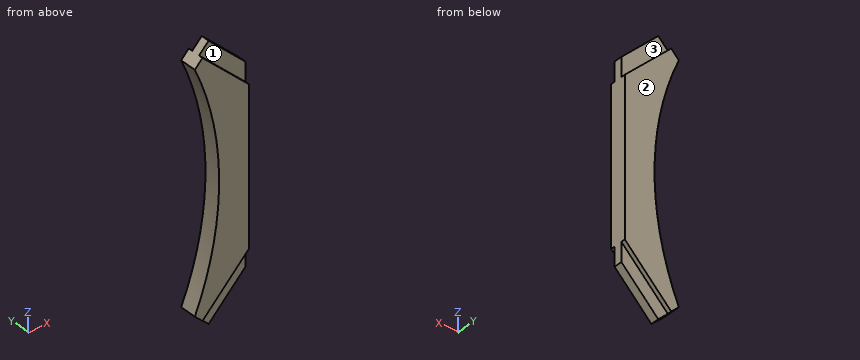
```python
from build123d import *

# Parameters (mm, degrees)
F1_DEPTH = 38.1
F2_DEPTH = 19.05


with BuildPart() as f1:
    # F0 (on Front) → F1 (new body, symmetric)
    with BuildSketch(Plane.XZ):
        with BuildLine():
            Line((127, 289.350816), (-127, 543.350816))
            ThreePointArc((-127, 543.350816), (-12.7, -4.446916), (-127, -552.244648))
            Line((-127, -552.244648), (127, -298.244648))
            Line((127, -298.244648), (127, 289.350816))
        make_face()
        Polygon((127, -298.244648), (-127, -552.244648), (-100.059232, -579.185416), (127, -352.126184), align=None)
        Polygon((-100.059232, 570.291584), (-127, 543.350816), (127, 289.350816), (127, 343.232352), align=None)
        Polygon((-91.078976, 579.27184), (-100.059232, 570.291584), (127, 343.232352), (127, 361.192865), align=None)
        Polygon((127, -352.126184), (-100.059232, -579.185416), (-91.078976, -588.165672), (127, -370.086696), align=None)
    extrude(amount=F1_DEPTH, both=True)

    # F0 (on Front) → F2 (join, symmetric)
    with BuildSketch(Plane.XZ):
        Polygon((127, 361.192865), (127, 450.995426), (-46.177695, 624.173121), (-91.078976, 579.27184), align=None)
        Polygon((127, -370.086696), (-91.078976, -588.165672), (-46.177695, -633.066953), (127, -459.889258), align=None)
    extrude(amount=F2_DEPTH, both=True)


solid = f1.part
```
Source: CAD feature listing. Evaluate the final solid. Frame: model axes, mm. Face numbers are marked on the shaded views. A direction names the side the tool comes from. Round coordinates to 2 decimals unless told otherwise and drop trailing zeros. Write each loop counter-clockwise with the first axis right and the second up, starting at its lowest first coordinate (ties: lowest second). Pieces come first, ordered by that corner, then holes. Notation, with made-up numbers: M 88.25,3 L 130.25,3 A23 cw 130.25,27 Z; hole C 53.5,24.5 d11. An arc over 180 degrees is marked long. Answer as a JSON object with one key per item and string values. Group by question number.
(1) Section query B-B on y = -8. Output: boundary loops of the cut face in (x, z).
(2) First-contact query: pin 1 (12 mm diameter, centred on y = 2.5, z = 291, fed in from -X); pin 2 (2 mm diameter, centred on x = 97.5, z = -449.5, fed in from +Y); pin 3 (3 mm diameter, centred on x = 87, y = -29.5, fed in from +Z). Flat tips, straight axial feed; report the tip coordinate or a pass-through.
(3) Section query D-D on x = 60. Output: boundary loops of the cut face in (y, z).
(4) Reachability of the marked faces 1, 2 and 3 from +Z, -Z, +X, -X, +Y, -Y: full face, straight path, thin tool, end or side. Return the list, or none.
(5) Section query A-A on x = -73.5. Output: boundary loops of the cut face in (y, z), then the cut area to 3 significant figures.
(6) Section query C-C on z = -532.5. Output: boundary loops of the cut face in (x, y).
(7) Ray query, line 1 (X direction, y = -17.5, z = -23); line 2 (Z direction, x = 34, y = -22); line 3 (X direction, y = -31, z = 145). Return the intervals inside material, ascending. Write a range as [from, to].
Computed values:
{
 "1": {"outline": "M -127,-552.24 L -46.18,-633.07 L 127,-459.89 L 127,451 L -46.18,624.17 L -127,543.35 A1369.85 cw Z"},
 "2": {"pin 1": "x = -46.28", "pin 2": "y = 19.05", "pin 3": "z = 402.69"},
 "3": {"outline": "M -38.1,-437.09 L -19.05,-437.09 L -19.05,-526.89 L 19.05,-526.89 L 19.05,-437.09 L 38.1,-437.09 L 38.1,428.19 L 19.05,428.19 L 19.05,518 L -19.05,518 L -19.05,428.19 L -38.1,428.19 Z"},
 "4": {"face 1": "+Z, +X, -Y", "face 2": "+Z, -Z, +X, -X, +Y", "face 3": "+Z, +X, +Y"},
 "5": {"outline": "M -38.1,-570.59 L -19.05,-570.59 L -19.05,-605.74 L 19.05,-605.74 L 19.05,-570.59 L 38.1,-570.59 L 38.1,-408.03 L -38.1,-408.03 Z; M -38.1,399.13 L 38.1,399.13 L 38.1,561.69 L 19.05,561.69 L 19.05,596.85 L -19.05,596.85 L -19.05,561.69 L -38.1,561.69 Z", "area": "27,500 mm^2"},
 "6": {"outline": "M -118.57,-38.1 L -35.41,-38.1 L -35.41,-19.05 L 54.39,-19.05 L 54.39,19.05 L -35.41,19.05 L -35.41,38.1 L -118.57,38.1 Z"},
 "7": {"line 1": "[-12.83, 127]", "line 2": "[-463.09, 454.19]", "line 3": "[-20.88, 127]"}
}
